For this review, take the finished solid that the model builds, in its own axes (mm). Face numbers are marked on the shaded views. A direction names the side the tool comes from. Give positions to 0.01 mm unless a question says otherwise; leave off trailing zeros. Write each loop counter-clockwise with the first axis right and the second up, starting at its lowest first coordinate (ties: lowest second). Pieces come first, ordered by that corner, then holes. Notation, with made-up numbers: (11, -9) -> (31, -9) arc R22 ccw to (31, -3) -> close; hole circle Ø10 at (0, -26). An arc over 180 degrees is marked (long way). Write item = value, one per line.
```python
from build123d import *

# Parameters (mm, degrees)
F2_R     = 3.4798
F3_DEPTH = 6.35
F4_SIZE2 = 0.6096
F4_SIZE  = 0.6096


# Not quite as in the source:
# - a variable given as a bare number and used for a length is read in inches; the dataset says mm whatever the document's units were


with BuildPart() as f3:
    # F2 (on Top) → F3 (new body)
    with BuildSketch(Plane.XY):
        with BuildLine():
            ThreePointArc((-3.81, -5.08), (-5.6796126628, -2.8398063314), (-6.35, 0))
            Line((-6.35, 0), (-6.35, -63.5))
            ThreePointArc((-6.35, -63.5), (-5.6796126628, -60.6601936686), (-3.81, -58.42))
            Line((-3.81, -58.42), (-3.81, -5.08))
        make_face()
        with BuildLine():
            ThreePointArc((3.81, -5.08), (5.6796126628, -2.8398063314), (6.35, 0))
            ThreePointArc((6.35, 0), (0, 6.35), (-6.35, 0))
            ThreePointArc((-6.35, 0), (-5.6796126628, -2.8398063314), (-3.81, -5.08))
            ThreePointArc((-3.81, -5.08), (0, -6.35), (3.81, -5.08))
        make_face()
        Circle(F2_R, mode=Mode.SUBTRACT)
        with BuildLine():
            Line((6.35, -63.5), (6.35, 0))
            ThreePointArc((6.35, 0), (5.6796126628, -2.8398063314), (3.81, -5.08))
            Line((3.81, -5.08), (3.81, -58.42))
            ThreePointArc((3.81, -58.42), (5.6796126628, -60.6601936686), (6.35, -63.5))
        make_face()
        with BuildLine():
            ThreePointArc((-6.35, -63.5), (0, -69.85), (6.35, -63.5))
            ThreePointArc((6.35, -63.5), (5.6796126628, -60.6601936686), (3.81, -58.42))
            ThreePointArc((3.81, -58.42), (0, -57.15), (-3.81, -58.42))
            ThreePointArc((-3.81, -58.42), (-5.6796126628, -60.6601936686), (-6.35, -63.5))
        make_face()
        with Locations((0, -63.5)):
            Circle(F2_R, mode=Mode.SUBTRACT)
    extrude(amount=F3_DEPTH)

    # F4
    f4_edges = [f3.edges().sort_by_distance(p)[0] for p in [
        (-3.4798, 0, 6.35),
        (-3.4798, -63.5, 6.35),
        (-3.4798, 0, 0),
        (-3.4798, -63.5, 0),
    ]]
    chamfer(f4_edges, length=F4_SIZE, length2=F4_SIZE2)


solid = f3.part
```
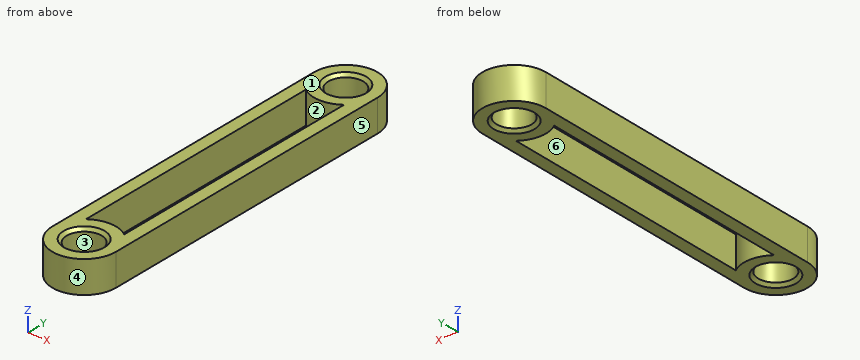
(1) Tool access review of the marked faces 5 and 6: name each direction out of +Z, -Z, +X, -X, +Y, -Y from which nothing blocks a thin tool from reaching the whole face with its end or side.
Answers below:
face_5 = +Z, -Z, +X, +Y, -Y
face_6 = +Z, -Z
(2) The part is to be moulded in two halves that separate along X. For the marked faces 1, 2, 3 and 4, say which applies: released by +X, released by -X, zero draft, split by the parting line, or undercut.
Answers below:
face_1 = zero draft
face_2 = undercut
face_3 = undercut
face_4 = split by the parting line
(3) For pin 1 (2 mm diameter, centred on x = -4, z = 3.5, fed in from -Y); pin 2 (2 mm diameter, centred on x = 5, z = 4, fed in from -Y); pin 3 (5.5 mm diameter, centred on x = 0, y = -63.5, fed in from +Z), all flat-tipped, find the tip position at first contact; note any pin that passes through.
Answers below:
pin_1 = -69.1
pin_2 = -68.43
pin_3 = through
(4) To check wall thickness, follow probe 1 along Y at (x, z) = (0, 3.05); probe 2 along X at (y, z) = (-28, 3.5); probe 3 along Y at (x, z) = (0.5, 2.5). State the ranges of each line that lie inside material, in increasing order.
Answers below:
probe_1 = -69.85 to -66.98, -60.02 to -57.15, -6.35 to -3.48, 3.48 to 6.35
probe_2 = -6.35 to -3.81, 3.81 to 6.35
probe_3 = -69.83 to -66.94, -60.06 to -57.17, -6.33 to -3.44, 3.44 to 6.33
(5) Take a section at B-B (z = 3.5). Write out the cut boundary in (x, y).
Answers below:
outline = (-6.35, -63.5) arc R6.35 ccw to (6.35, -63.5) -> (6.35, 0) arc R6.35 ccw to (-6.35, 0) -> close; hole (-3.81, -58.42) arc R6.35 cw to (3.81, -58.42) -> (3.81, -5.08) arc R6.35 cw to (-3.81, -5.08) -> close; hole circle Ø6.96 at (0, -63.5); hole circle Ø6.96 at (0, 0)
(6) Take a section at A-A (x = 0). Write out the cut boundary in (y, z).
Answers below:
outline = (-69.85, 0) -> (-67.59, 0) -> (-66.98, 0.61) -> (-66.98, 5.74) -> (-67.59, 6.35) -> (-69.85, 6.35) -> close; (-60.02, 0.61) -> (-59.41, 0) -> (-57.15, 0) -> (-57.15, 6.35) -> (-59.41, 6.35) -> (-60.02, 5.74) -> close; (-6.35, 0) -> (-4.09, 0) -> (-3.48, 0.61) -> (-3.48, 5.74) -> (-4.09, 6.35) -> (-6.35, 6.35) -> close; (3.48, 0.61) -> (4.09, 0) -> (6.35, 0) -> (6.35, 6.35) -> (4.09, 6.35) -> (3.48, 5.74) -> close
